from build123d import *

# Parameters (mm, degrees)
SZKIC1_R                    = 9
DODANIE_WYCI_GNI_CIE1_DEPTH = 25
SZKIC2_R                    = 4
WYTNIJ_WYCI_GNI_CIE1_DEPTH  = 10
SZKIC3_R                    = 2.5
WYTNIJ_WYCI_GNI_CIE2_DEPTH  = 10
SFAZOWANIE1_SIZE            = 0.5


with BuildPart() as part:
    # Szkic1 → Dodanie-wyciągnięcie1 (new body)
    with BuildSketch(Plane.XY):
        Circle(SZKIC1_R)
    extrude(amount=DODANIE_WYCI_GNI_CIE1_DEPTH)

    # Szkic2 → Wytnij-wyciągnięcie1 (cut)
    with BuildSketch(Plane.XY.offset(25)):
        Circle(SZKIC2_R)
    extrude(amount=-WYTNIJ_WYCI_GNI_CIE1_DEPTH, mode=Mode.SUBTRACT)

    # Szkic3 → Wytnij-wyciągnięcie2 (cut)
    with BuildSketch(Plane(origin=(0, 0, 0), x_dir=(-1, 0, 0), z_dir=(0, 0, -1))):
        Circle(SZKIC3_R)
    extrude(amount=-WYTNIJ_WYCI_GNI_CIE2_DEPTH, mode=Mode.SUBTRACT)

    # Sfazowanie1
    sfazowanie1_edges = [part.edges().sort_by_distance(p)[0] for p in [
        (2.5, 0, 0),
        (-9, 0, 0),
        (-9, 0, 25),
        (-4, 0, 25),
    ]]
    chamfer(sfazowanie1_edges, length=SFAZOWANIE1_SIZE)


solid = part.part
Build history of the part. All positions in model axes, mm. A direction names the side the tool comes from. Give positions to 0.01 mm unless a question says otherwise; leave off trailing zeros. Order: outer loops, then holes, each group sorted by start corner. A loop starts at its lowest first (then second) coordinate and runs counter-clockwise, first axis right, second up. Notation, with made-up numbers: M -37.75,-22.5 L 15.25,-22.5 A16 cw 15.25,-12.5 Z; hole C 3,5.5 d2. An arc over 180 degrees is marked long. Put each result on its own line as item: value.
Item 1: Slice it at C-C, the plane z = 2.25. Write the cut outline in (x, y), plus the area to 3 significant figures.
From the geometry:
outline: C 0,0 d18; hole C 0,0 d5
area: 235 mm2
Item 2: 3-axis set-ups, long thin cutter, end or side, ignore diameter. For faces 1 (the cylindrical face through (-0.867, -3.905, 19.816)), 2 (the flat face through (0, 0, 10)), 3 (the flat face through (4, -4, 25)): which of +Z, -Z, +X, -X, +Y, -Y reach the whole face in a straight line?
From the geometry:
face 1: +Z
face 2: -Z
face 3: +Z, +X, -X, +Y, -Y
Item 3: Two-plate mould, pull along X, no slides. Class faces 4 (the cylindrical face through (0.54, -2.44, 5.18)), 5 (the cylindrical face through (-1.172, 8.923, 12.332)), 6 (the flat face through (4, 0, 0)), 7 (the flat face through (0, 0, 15)): +X half, -X half, draft (parallel to the pull), parting line (faces both ways), or undercut.
From the geometry:
face 4: undercut
face 5: parting line
face 6: draft
face 7: undercut
Item 4: Slice it at A-A, the plane x = 0. Write the cut outline in (y, z).
From the geometry:
outline: M -9,0.5 L -8.5,0 L -3,0 L -2.5,0.5 L -2.5,10 L 2.5,10 L 2.5,0.5 L 3,0 L 8.5,0 L 9,0.5 L 9,24.5 L 8.5,25 L 4.5,25 L 4,24.5 L 4,15 L -4,15 L -4,24.5 L -4.5,25 L -8.5,25 L -9,24.5 Z
Item 5: Probe line 1 (Y direction, x = 0, z = 6); line 2 (Y direction, x = 0, z = 19.25); line 3 (Z direction, x = 0.75, y = -1.5). List the from-to ranges inside material, lowest first. Write a range as [from, to].
From the geometry:
line 1: y = [-9, -2.5], [2.5, 9]
line 2: y = [-9, -4], [4, 9]
line 3: z = [10, 15]
Item 6: Flat gauge pins, fed straight in: pin 1 Ø3 at (x, z) = (-2, 17.5) entering from -Y; pin 2 Ø1.5 at (x, y) = (3.5, -2) entering from -Z; pin 3 Ø1.5 at (x, y) = (-0.5, 0) entering from -Z; pin 4 Ø2 at (y, z) = (-6, 19) entering from +X. Where does each tip first touch, or does it go through?
From the geometry:
pin 1: stops at y = -8.99
pin 2: stops at z = 0
pin 3: stops at z = 10
pin 4: stops at x = 7.48
Item 7: Slice it at D-D, the plane z = 11.75. Write the cut outline in (x, y).
From the geometry:
outline: C 0,0 d18
